Could you check a few things on this model? Use its own coordinates, in mm. Give positions to 0.01 mm unless a question says otherwise; leave off trailing zeros. Write each loop counter-clockwise with the first axis right and the second up, starting at its lowest first coordinate (ties: lowest second). Pieces come first, ordered by that corner, then holes. Notation, with made-up numbers: (29.5, -29.75) - (59.5, -29.75) arc R28 ccw to (59.5, 1.25) - close; hole circle Ø6 at (51, -22.75). An arc over 180 degrees is marked (long way). Write item = value, one per line.
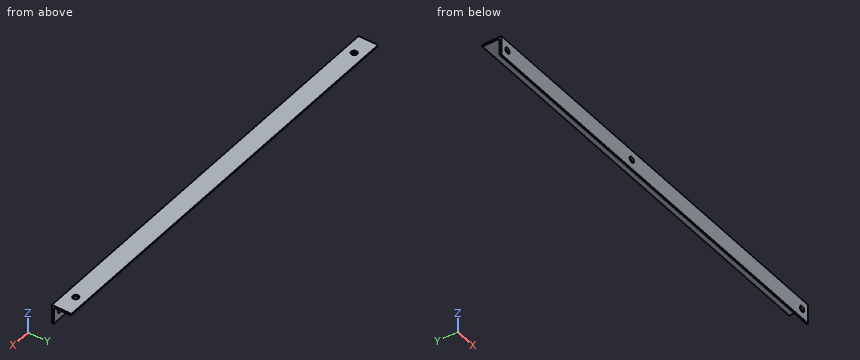
from build123d import *

# Parameters (mm, degrees)
EXTRUDE_1_DEPTH     = 434
SKETCH_2_R          = 3
CUT_EXTRUDE_1_DEPTH = 435.920682424
SKETCH_3_R          = 3
CUT_EXTRUDE_2_DEPTH = 435.833301393
SKETCH_5_R          = 3
CUT_EXTRUDE_4_DEPTH = 2


with BuildPart() as part:
    # Эскиз1 → Бобышка-Вытянуть1 (new body)
    with BuildSketch(Plane(origin=(0, 0, 0), x_dir=(0, 0, -1), z_dir=(1, 0, 0))):
        with BuildLine():
            Line((0, 0), (0, 20))
            Line((0, 20), (1, 20))
            ThreePointArc((1, 20), (1.707106781, 19.707106781), (2, 19))
            Line((2, 19), (2, 3))
            ThreePointArc((2, 3), (2.292893219, 2.292893219), (3, 2))
            Line((3, 2), (19, 2))
            ThreePointArc((19, 2), (19.707106781, 1.707106781), (20, 1))
            Line((20, 1), (20, 0))
            Line((20, 0), (0, 0))
        make_face()
    extrude(amount=EXTRUDE_1_DEPTH)

    # Эскиз2 → Вырез-Вытянуть1 (cut, through all)
    with BuildSketch(Plane.XZ):
        with Locations(Location((425.5, -10, 0), (0, 0, 270))):
            Circle(SKETCH_2_R)
        with Locations(Location((8.5, -10, 0), (0, 0, 270))):
            Circle(SKETCH_2_R)
    extrude(amount=-CUT_EXTRUDE_1_DEPTH, mode=Mode.SUBTRACT)

    # Эскиз3 → Вырез-Вытянуть2 (cut, through all)
    with BuildSketch(Plane(origin=(0, 0, -2), x_dir=(-1, 0, 0), z_dir=(0, 0, -1))):
        with Locations(Location((-414, 10, 0), (0, 0, 90))):
            Circle(SKETCH_3_R)
        with Locations(Location((-20, 10, 0), (0, 0, 90))):
            Circle(SKETCH_3_R)
    extrude(amount=-CUT_EXTRUDE_2_DEPTH, mode=Mode.SUBTRACT)

    # Эскиз5 → Вырез-Вытянуть4 (cut)
    with BuildSketch(Plane(origin=(0, 2, 0), x_dir=(1, 0, 0), z_dir=(0, 1, 0))):
        with Locations(Location((184.5, 10, 0), (0, 0, 270))):
            Circle(SKETCH_5_R)
    extrude(amount=-CUT_EXTRUDE_4_DEPTH, mode=Mode.SUBTRACT)


solid = part.part
1. If we section it at B-B, the plane x = 55: Please give me the cut outline in (y, z).
Filled sheet:
outline = (0, -20) - (1, -20) arc R1 ccw to (2, -19) - (2, -3) arc R1 cw to (3, -2) - (19, -2) arc R1 ccw to (20, -1) - (20, 0) - (0, 0) - close
2. If we section it at C-C, the plane y = 16: Please give me the cut outline in (x, z), and give its area (3 significant figures).
Filled sheet:
outline = (0, -2) - (434, -2) - (434, 0) - (0, 0) - close
area = 868 mm2
3. I need wall thicknesses on line 1 (X direction, y = 1.3, z = -10); line 2 (X direction, y = 10, z = -1.2); line 3 (Z direction, x = 184.5, y = 0.55). Which ranges of each line are inside material? Lowest first, please.
Filled sheet:
line_1 = 0 to 5.5, 11.5 to 181.5, 187.5 to 422.5, 428.5 to 434
line_2 = 0 to 17, 23 to 411, 417 to 434
line_3 = -20 to -13, -7 to 0
4. If we section it at A-A, the plane z = -10: Please give me the cut outline in (x, y), and give its area (3 significant figures).
Filled sheet:
outline = (0, 0) - (5.5, 0) - (5.5, 2) - (0, 2) - close; (11.5, 0) - (181.5, 0) - (181.5, 2) - (11.5, 2) - close; (187.5, 0) - (422.5, 0) - (422.5, 2) - (187.5, 2) - close; (428.5, 0) - (434, 0) - (434, 2) - (428.5, 2) - close
area = 832 mm2
5. For pin 1 (3 mm diameter, centred on x = 322.5, y = 16, fed in from +Z); pin 2 (12 mm diameter, centred on x = 291, y = 16, fed in from -Z); pin 3 (12 mm diameter, centred on x = 311.5, z = -10.5, fed in from +Y), each with a flat end and sliding along its axis, tell me the tip position at first contact or that it passes through.
Filled sheet:
pin_1 = 0
pin_2 = -2
pin_3 = 2
